```python
from build123d import *

# Parameters (mm, degrees)
F0_R          = 53.3590641314
F1_DEPTH      = 2.54
F2_R          = 53.3590641314
F2_R_2        = 50.8190641314
F3_DEPTH      = 25.4
F5_R          = 4.731473746
F6_DEPTH      = 53.3600641314
F6_DEPTH_BACK = 53.3600641314


# Not quite as in the source:
# - a fillet or chamfer that OpenCascade refuses, or shapes differently, is made with other operations: its cross-section is extruded or revolved along the edge and cut away or added


with BuildPart() as f1:
    # F0 (on Front) → F1 (new body)
    with BuildSketch(Plane.XZ):
        Circle(F0_R)
    extrude(amount=F1_DEPTH)

    # F2 (on face) → F3 (join)
    with BuildSketch(Plane.XZ.offset(2.54)):
        Circle(F2_R)
        Circle(F2_R_2, mode=Mode.SUBTRACT)
    extrude(amount=F3_DEPTH)

    # F4: fillet of radius 5.08 on 1 edges, made by hand

    # F4_s1 → F4_t2 (revolve, cut)
    with BuildSketch(Plane.XY):
        with BuildLine():
            ThreePointArc((53.3588640934, -27.9403463882), (51.4992986538, -26.0804748362), (50.8186641314, -23.5400334454))
            Line((50.8186641314, -23.5400334454), (50.3105275628, -23.5400334454))
            ThreePointArc((50.3105275628, -23.5400334454), (50.3109275628, -25.7400167227), (50.3109275628, -27.94))
            Line((50.3109275628, -27.94), (50.8190641314, -28.4481365685))
            ThreePointArc((50.8190641314, -28.4481365685), (52.0889641124, -28.4481365685), (53.104747521, -28.3803776825))
            Line((53.104747521, -28.3803776825), (53.3588640934, -27.9403463882))
        make_face()
    revolve(axis=Axis((0, -27.94, 0), (0, -1, 0)), mode=Mode.SUBTRACT)

    # F5 (on Top) → F6 (cut, two sides)
    with BuildSketch(Plane.XY) as f6_sk:
        with Locations((0, -28.3043142408)):
            Circle(F5_R)
    extrude(amount=-F6_DEPTH, mode=Mode.SUBTRACT)
    extrude(f6_sk.sketch, amount=F6_DEPTH_BACK, mode=Mode.SUBTRACT)


solid = f1.part
```
Input: part model. Units: mm. Frame: model coordinates. A direction names the side the tool comes from. Give positions to 0.01 mm unless a question says otherwise; leave off trailing zeros. Order: outer loops, then holes, each group sorted by start corner. A loop starts at its lowest first (then second) coordinate and runs counter-clockwise, first axis right, second up.
1. Set-up query: faces 1 (the face through (-1, -2.54, 1)), 2 (the face through (0.099, -23.574, 52.061)). Return all of +Z, -Z, +X, -X, +Y, -Y with unobstructed straight access to the full face (end or side cutting, diameter ignored); none if empty.
Computed:
face 1: -Y
face 2: +Z, -Z, -Y
2. Line query: probe 1 along Z at (x, y) = (0, -12.5); probe 2 along Y at (x, z) = (11.5, 41). Output: solid intervals per line, ascending.
Computed:
probe 1: z = -53.36 to -50.82, 50.82 to 53.36
probe 2: y = -2.54 to 0
3. Cut plane A-A (y = -15). Return loops of the section in (x, z).
Computed:
outline: circle Ø106.72 at (0, 0); hole circle Ø101.64 at (0, 0)
4. Pin query (flat end, axial travel): pin 1 Ø4 at (x, z) = (1.5, 30) entering from -Y; pin 2 Ø1 at (y, z) = (-16.5, 20.5) entering from +X; pin 3 Ø3 at (x, y) = (6, -19.5) entering from -Z. Return the tip coordinate at first contact, or that it passes through.
Computed:
pin 1: stops at y = -2.54
pin 2: stops at x = 49.47
pin 3: stops at z = -53.17
